```python
from build123d import *

# Parameters (mm, degrees)
EXTRUDE1_DEPTH = 7.5
SKETCH2_R      = 1.8
EXTRUDE2_DEPTH = 6
SKETCH_R       = 1.8
EXTRUDE3_DEPTH = 3
FILLET1_R      = 1
CHAMFER1_SIZE  = 0.25


with BuildPart() as part:
    # Sketch1 → Extrude1 (new body)
    with BuildSketch(Plane.XY):
        with BuildLine():
            Line((-2.15, 0), (-2.15, 1))
            ThreePointArc((-2.15, 1), (0, 3.15), (2.15, 1))
            Line((2.15, 1), (2.15, 0))
            Line((2.15, 0), (10.5, 0))
            Line((10.5, 0), (10.5, 5))
            Line((10.5, 5), (-10.5, 5))
            Line((-10.5, 5), (-10.5, 0))
            Line((-10.5, 0), (-2.15, 0))
        make_face()
    extrude(amount=EXTRUDE1_DEPTH)

    # Sketch2 → Extrude2 (cut, through all)
    with BuildSketch(Plane(origin=(0, 5, 0), x_dir=(1, 0, 0), z_dir=(0, 1, 0))):
        with Locations((-6.5, -3.75)):
            Circle(SKETCH2_R)
        with Locations((6.5, -3.75)):
            Circle(SKETCH2_R)
    extrude(amount=-EXTRUDE2_DEPTH, mode=Mode.SUBTRACT)

    # Sketch → Extrude3 (cut)
    with BuildSketch(Plane(origin=(0, 5, 0), x_dir=(1, 0, 0), z_dir=(0, 1, 0))):
        Polygon((-8.116580754, -6.55), (-9.733161507, -3.75), (-8.116580754, -0.95), (-4.883419246, -0.95), (-3.266838493, -3.75), (-4.883419246, -6.55), align=None)
        with Locations((-6.5, -3.75)):
            Circle(SKETCH_R, mode=Mode.SUBTRACT)
        Polygon((9.733161507, -3.75), (8.116580754, -0.95), (4.883419246, -0.95), (3.266838493, -3.75), (4.883419246, -6.55), (8.116580754, -6.55), align=None)
        with Locations((6.5, -3.75)):
            Circle(SKETCH_R, mode=Mode.SUBTRACT)
    extrude(amount=-EXTRUDE3_DEPTH, mode=Mode.SUBTRACT)

    # Fillet1
    fillet1_edges = [part.edges().sort_by_distance(p)[0] for p in [
        (10.5, 2.5, 7.5),
        (-10.5, 2.5, 7.5),
        (-10.5, 2.5, 0),
        (10.5, 2.5, 0),
    ]]
    fillet(fillet1_edges, radius=FILLET1_R)

    # Chamfer1
    chamfer1_edges = [part.edges().sort_by_distance(p)[0] for p in [
        (5.825, 0, 7.5),
        (-8.3, 0, 3.75),
        (4.7, 0, 3.75),
        (10.5, 0, 3.75),
        (-5.825, 0, 0),
        (10.207106781, 0, 7.207106781),
        (10.207106781, 0, 0.292893219),
        (-5.825, 0, 7.5),
        (-10.5, 0, 3.75),
        (-10.207106781, 0, 7.207106781),
        (-10.207106781, 0, 0.292893219),
        (5.825, 0, 0),
    ]]
    chamfer(chamfer1_edges, length=CHAMFER1_SIZE)


solid = part.part
```
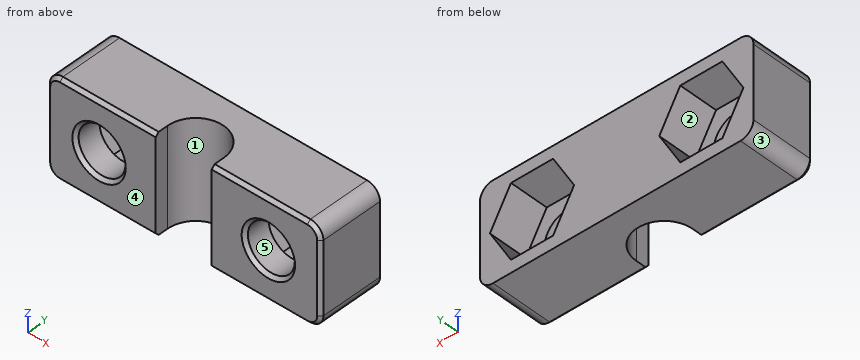
Geometry: final body of the model. Coordinates: model frame, mm. Face numbers are marked on the shaded views. A direction names the side the tool comes from. Round coordinates to 2 decimals unless told otherwise and drop trailing zeros. Order: outer loops, then holes, each group sorted by start corner. A loop starts at its lowest first (then second) coordinate and runs counter-clockwise, first axis right, second up. Notation, with made-up numbers: (73, -30) -> (112, -30) arc R27 cw to (112, -8) -> close; hole circle Ø9 at (86, -35.5). An arc over 180 degrees is marked (long way). Write each question's results on one line, items separated by ' | '.
Q1. Section query C-C (x = -3.5). Output: boundary loops of the cut face in (y, z).
Response values:
outline: (0, 0.25) -> (0.25, 0) -> (5, 0) -> (5, 3.35) -> (2, 3.35) -> (2, 4.15) -> (5, 4.15) -> (5, 7.5) -> (0.25, 7.5) -> (0, 7.25) -> close
Q2. Section query A-A (x = 6.5). Output: boundary loops of the cut face in (y, z), and give its area (3 significant figures).
Response values:
outline: (0, 0.25) -> (0.25, 0) -> (5, 0) -> (5, 0.95) -> (2, 0.95) -> (2, 1.95) -> (0.25, 1.95) -> (0, 1.7) -> close; (0, 5.8) -> (0.25, 5.55) -> (2, 5.55) -> (2, 6.55) -> (5, 6.55) -> (5, 7.5) -> (0.25, 7.5) -> (0, 7.25) -> close | area: 13.4 mm²
Q3. Pull-direction query (X, two-part tool) for the marked faces 3, 4 and 5; classes: released by +X, released by -X, zero draft, split by the parting line, or undercut.
Response values:
face 3: released by -X | face 4: zero draft | face 5: undercut
Q4. Pin query (flat end, axial travel): pin 1 Ø3 at (x, z) = (-8, 3) entering from +Y; pin 2 Ø2 at (x, z) = (-6.5, 3.75) entering from +Y; pin 3 Ø3 at (x, z) = (5.5, 4.5) entering from +Y. Return the tip coordinate at first contact, or that it passes through.
Response values:
pin 1: y = 5 | pin 2: through | pin 3: y = 2
Q5. Ray query, line 1 along X through (y, z) = (0.85, 3.75); line 2 along Z through (x, y) = (6.5, 1.6). Return the intervals inside material, ascending.
Response values:
line 1: -10.5 to -8.3, -4.7 to -2.15, 2.15 to 4.7, 8.3 to 10.5 | line 2: 0 to 1.95, 5.55 to 7.5
Q6. Access query for the marked faces 1 and 2. Directions: +Z, -Z, +X, -X, +Y, -Y. A direction counts if a zero-diameter tool reaches every point of the face in a straight line with its end or side. Return the directions, or none.
Response values:
face 1: +Z, -Z, -Y | face 2: +Y
Q7. Section query B-B (y = 3.5). Output: boundary loops of the cut face in (x, z).
Response values:
outline: (-10.5, 1) arc R1 ccw to (-9.5, 0) -> (9.5, 0) arc R1 ccw to (10.5, 1) -> (10.5, 6.5) arc R1 ccw to (9.5, 7.5) -> (-9.5, 7.5) arc R1 ccw to (-10.5, 6.5) -> close; hole (-9.73, 3.75) -> (-8.12, 0.95) -> (-4.88, 0.95) -> (-3.27, 3.75) -> (-4.88, 6.55) -> (-8.12, 6.55) -> close; hole (3.27, 3.75) -> (4.88, 0.95) -> (8.12, 0.95) -> (9.73, 3.75) -> (8.12, 6.55) -> (4.88, 6.55) -> close
Q8. Section query D-D (x = 0.25). Output: boundary loops of the cut face in (y, z).
Response values:
outline: (3.14, 0) -> (5, 0) -> (5, 7.5) -> (3.14, 7.5) -> close
